```python
from build123d import *

# Parameters (mm, degrees)
BOSS_EXTRU_1_DEPTH      = 60
ESQUISSE2_W             = 10
ESQUISSE2_H             = 70.243389495
ENL_V_MAT_EXTRU_1_DEPTH = 10


with BuildPart() as part:
    # Esquisse1 → Boss.-Extru.1 (new body)
    with BuildSketch(Plane.XY):
        Polygon((0, 0), (50, 0), (50, 9), (50, 18), (0, 18), align=None)
    extrude(amount=BOSS_EXTRU_1_DEPTH)

    # Esquisse2 → Enlèv. mat.-Extru.1 (cut)
    with BuildSketch(Plane(origin=(0, 18, 0), x_dir=(1, 0, 0), z_dir=(0, 1, 0))):
        with Locations((15, -30.175170548)):
            Rectangle(ESQUISSE2_W, ESQUISSE2_H)
        with Locations((35, -30.175170548)):
            Rectangle(ESQUISSE2_W, ESQUISSE2_H)
    extrude(amount=-ENL_V_MAT_EXTRU_1_DEPTH, mode=Mode.SUBTRACT)


solid = part.part
```
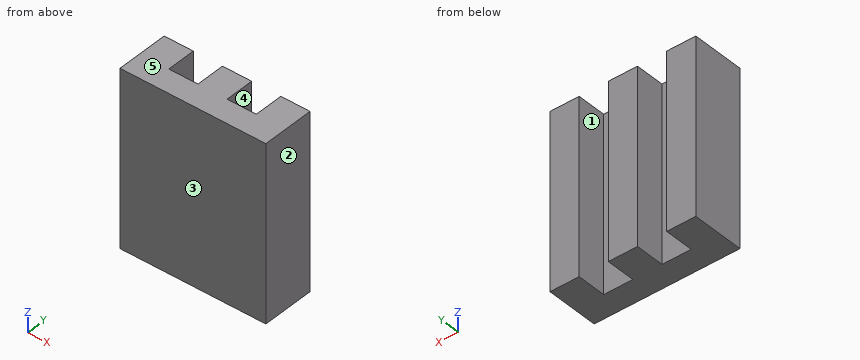
Work out the finished part from the listing and answer in its coordinate system (mm). Face numbers are marked on the shaded views. A direction names the side the tool comes from. Give positions to 0.01 mm unless a question says otherwise; leave off trailing zeros. Loops run counter-clockwise (first coordinate to the right, second up) from the corner with the lowest first, then second, coordinate; pieces in that order, holes last. Notation, with made-up numbers: (4, -20.75) -> (36, -20.75) arc R23 cw to (36, 2.25) -> close; hole circle Ø2 at (72.25, -28.75). An arc over 180 degrees is marked (long way). One line per question, with ' | ' between items. Start each with the question number.
1) Each of these flat-tipped pins is pushed along its axis until it touches: pin 1 (5 mm diameter, centred on y = 12.5, z = 42, fed in from -X); pin 2 (3 mm diameter, centred on x = 13, z = 17, fed in from +Y). Where does it stop, or does it pass through?
2) For the marked faces 4 and 5, determine the directions among +Z, -Z, +X, -X, +Y, -Y from which every point of the face is accessible in a straight line to the end or side of a thin tool.
3) Section C-C, the plane x = 18 is taken. Determine the outline of the cut face in (y, z).
4) Section B-B, the plane z = 15.5 is taken. Determine the outline of the cut face in (x, y), then the cut area to 3 significant figures.
5) Straight lines are drawn through the part: L1, parallel to X at y = 17, z = 10.5; L2, parallel to Y at x = 33, z = 26.5. For each, find the intervals that lie inside material, in ascending order.
6) Determine the mould class of the marked faces 1, 2 and 3 for opening direction X: +X half, -X half, draft (parallel to the pull), parting line (faces both ways), or undercut.
7) Section A-A, the plane y = 15.5 is taken. Determine the outline of the cut face in (x, z).
Resolved:
1) pin 1: x = 0 | pin 2: y = 8
2) face 4: +Z, -Z, +Y | face 5: +Z, +X, -X, +Y, -Y
3) outline: (0, 0) -> (8, 0) -> (8, 60) -> (0, 60) -> close
4) outline: (0, 0) -> (50, 0) -> (50, 18) -> (40, 18) -> (40, 8) -> (30, 8) -> (30, 18) -> (20, 18) -> (20, 8) -> (10, 8) -> (10, 18) -> (0, 18) -> close | area: 700 mm2
5) L1: 0 to 10, 20 to 30, 40 to 50 | L2: 0 to 8
6) face 1: undercut | face 2: +X half | face 3: draft
7) outline: (0, 0) -> (10, 0) -> (10, 60) -> (0, 60) -> close; (20, 0) -> (30, 0) -> (30, 60) -> (20, 60) -> close; (40, 0) -> (50, 0) -> (50, 60) -> (40, 60) -> close
